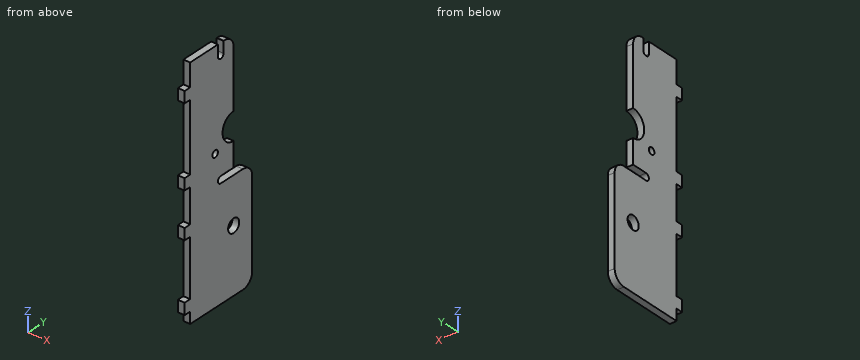
from build123d import *

# Parameters (mm, degrees)
SKETCH1_W           = 105
SKETCH1_H           = 23.5
BOSS_EXTRUDE1_DEPTH = 3
SKETCH2_R           = 6
SKETCH2_R_2         = 1.5
CUT_EXTRUDE1_DEPTH  = 4
CUT_EXTRUDE2_DEPTH  = 4
SKETCH4_W           = 3
SKETCH4_H           = 5
BOSS_EXTRUDE2_DEPTH = 3
CUT_EXTRUDE4_DEPTH  = 4
SKETCH5_W           = 3
SKETCH5_H           = 5
BOSS_EXTRUDE3_DEPTH = 3
SKETCH9_W           = 3
SKETCH9_H           = 48.5
BOSS_EXTRUDE5_DEPTH = 10
SKETCH10_R          = 3
CUT_EXTRUDE5_DEPTH  = 4
FILLET5_R           = 5


with BuildPart() as part:
    # Sketch1 → Boss-Extrude1 (new body)
    with BuildSketch(Plane(origin=(0, 0, 0), x_dir=(0, 0, -1), z_dir=(1, 0, 0))):
        with Locations((22.5, 11.75)):
            Rectangle(SKETCH1_W, SKETCH1_H)
    extrude(amount=BOSS_EXTRUDE1_DEPTH)

    # Sketch2 → Cut-Extrude1 (cut, through all)
    with BuildSketch(Plane(origin=(3, 0, 0), x_dir=(0, 0, -1), z_dir=(1, 0, 0))):
        with Locations((6.8, 23.5)):
            Circle(SKETCH2_R)
        with Locations((13.2, 13.5)):
            Circle(SKETCH2_R_2)
    extrude(amount=-CUT_EXTRUDE1_DEPTH, mode=Mode.SUBTRACT)

    # Sketch3 → Cut-Extrude2 (cut, through all)
    with BuildSketch(Plane(origin=(3, 0, 0), x_dir=(0, 0, -1), z_dir=(1, 0, 0))):
        with BuildLine():
            Line((-25, 15), (-30, 15))
            Line((-30, 15), (-30, 18))
            Line((-30, 18), (-25, 18))
            ThreePointArc((-25, 18), (-23.5, 16.5), (-25, 15))
        make_face()
    extrude(amount=-CUT_EXTRUDE2_DEPTH, mode=Mode.SUBTRACT)

    # Sketch4 → Boss-Extrude2 (add)
    with BuildSketch(Plane.XZ):
        with Locations((1.5, 17.5)):
            Rectangle(SKETCH4_W, SKETCH4_H)
    boss_extrude2 = extrude(amount=BOSS_EXTRUDE2_DEPTH)

    # Mirror4: Boss-Extrude2 across plane
    add(boss_extrude2.mirror(Plane.XY))

    # Sketch8 → Cut-Extrude4 (cut, through all)
    with BuildSketch(Plane(origin=(3, 0, 0), x_dir=(0, 0, -1), z_dir=(1, 0, 0))):
        with BuildLine():
            Line((23.5, 16.5), (23.5, 23.5))
            Line((23.5, 23.5), (26.5, 23.5))
            Line((26.5, 23.5), (26.5, 16.5))
            ThreePointArc((26.5, 16.5), (25, 15), (23.5, 16.5))
        make_face()
    extrude(amount=-CUT_EXTRUDE4_DEPTH, mode=Mode.SUBTRACT)

    # Sketch5 → Boss-Extrude3 (add)
    with BuildSketch(Plane.XZ):
        with Locations((1.5, -37.5)):
            Rectangle(SKETCH5_W, SKETCH5_H)
        with Locations((1.5, -67.5)):
            Rectangle(SKETCH5_W, SKETCH5_H)
    extrude(amount=BOSS_EXTRUDE3_DEPTH)

    # Sketch9 → Boss-Extrude5 (add)
    with BuildSketch(Plane(origin=(0, 23.5, 0), x_dir=(1, 0, 0), z_dir=(0, 1, 0))):
        with Locations((1.5, 50.75)):
            Rectangle(SKETCH9_W, SKETCH9_H)
    extrude(amount=BOSS_EXTRUDE5_DEPTH)

    # Sketch10 → Cut-Extrude5 (cut, through all)
    with BuildSketch(Plane(origin=(3, 0, 0), x_dir=(0, 0, -1), z_dir=(1, 0, 0))):
        with Locations((46.8, 23.5)):
            Circle(SKETCH10_R)
    extrude(amount=-CUT_EXTRUDE5_DEPTH, mode=Mode.SUBTRACT)

    # Fillet5
    fillet5_edges = [part.edges().sort_by_distance(p)[0] for p in [
        (1.5, 33.5, -26.5),
        (1.5, 33.5, -75),
        (1.5, 23.5, 30),
    ]]
    fillet(fillet5_edges, radius=FILLET5_R)


solid = part.part
Can you work these out from the model? Positions are in its coordinate system, mm. Coordinates: 2 decimals unless noted, no trailing zeros. Loops run counter-clockwise (first coordinate to the right, second up) from the corner with the lowest first, then second, coordinate; pieces in that order, holes last. Notation, with made-up numbers: (34, 40.25) - (78, 40.25) arc R15 cw to (78, 46.25) - close; hole circle Ø10 at (49, 74.25). An arc over 180 degrees is marked (long way). Answer as a JSON object with one key per item and string values. Group by question number.
Item 1: If I drill on L1, parallel to Y at x = 1.05, z = -46.8; L2, parallel to Y at x = 1.5, z = -13.2; L3, parallel to Y at x = 1.95, z = -7, over which ranges is the centre line in solid material (lowest first)? Write a range as from..to.
Item 2: For pin 1 (1.5 mm diameter, centred on x = 1.5, y = -2, fed in from -Z); pin 2 (2 mm diameter, centred on y = 22, z = 4, fed in from -X); pin 3 (0.9 mm diameter, centred on x = 1, z = -17, fed in from +Y); pin 4 (1.5 mm diameter, centred on x = 1.5, y = -2, fed in from +Z), each with a flat end and sliding along its axis, tell me the tip position at first contact or that it passes through.
Item 3: If we section it at C-C (z = -6.8): List the corners of the cut face in (x, y) for me.
Item 4: If we section it at A-A (z = -46.8): List the corners of the cut face in (x, y) for me.
Item 5: If we section it at B-B (x = 2.5): State how many separate pieces and enclosed holes the cut face has, plus the area to 3 significant figures.
Returned:
{
 "1": {"L1": "y = 0..20.5, 26.5..33.5", "L2": "y = 0..12, 15..23.5", "L3": "y = 0..17.5"},
 "2": {"pin 1": "stops at z = -70", "pin 2": "stops at x = 0", "pin 3": "stops at y = 23.5", "pin 4": "stops at z = 20"},
 "3": {"outline": "(0, 0) - (3, 0) - (3, 17.5) - (0, 17.5) - close"},
 "4": {"outline": "(0, 0) - (3, 0) - (3, 20.5) - (0, 20.5) - close; (0, 26.5) - (3, 26.5) - (3, 33.5) - (0, 33.5) - close"},
 "5": {"separate pieces": "1", "enclosed holes": "2", "area": "2,860 mm²"}
}
